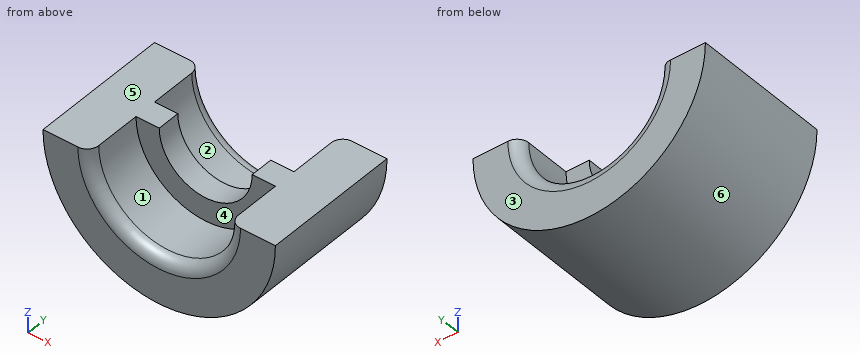
```python
from build123d import *

# Parameters (mm, degrees)
SKETCH1_W      = 1
SKETCH1_H      = 1
SKETCH1_W_2    = 2
SKETCH1_H_2    = 6
REVOLVE2_ANGLE = 180
FILLET3_R      = 0.5


with BuildPart() as part:
    # Sketch1 → Revolve2 (revolve)
    with BuildSketch(Plane.XY):
        with Locations((2.5, 0)):
            Rectangle(SKETCH1_W, SKETCH1_H)
        with Locations((4, 0)):
            Rectangle(SKETCH1_W_2, SKETCH1_H_2)
    revolve(axis=Axis((0, 0, 0), (0, 1, 0)), revolution_arc=REVOLVE2_ANGLE)

    # Fillet3
    fillet3_edges = [part.edges().sort_by_distance(p)[0] for p in [
        (0, 3, -3),
        (0, -3, -3),
    ]]
    fillet(fillet3_edges, radius=FILLET3_R)


solid = part.part
```
Can you work these out from the model? Positions are in its coordinate system, mm. Face numbers are marked on the shaded views. A direction names the side the tool comes from. Coordinates: 2 decimals unless noted, no trailing zeros. Loops run counter-clockwise (first coordinate to the right, second up) from the corner with the lowest first, then second, coordinate; pieces in that order, holes last. Notation, with made-up numbers: (76.25, -29.5) - (135.25, -29.5) arc R17 ccw to (135.25, -11.5) - close; hole circle Ø7 at (-32, 73.25). An arc over 180 degrees is marked (long way). Answer as CSV lines item,"result". Start each with the question number.
1) Thinking about a two-plate mould opening in X: for the marked faces 4, 5 and 6, which applies, pulls with the +X half, pulls with the -X half, needs draft (parallel to the pull), parting line crosses it, or undercut?
2) Suppose I cut it at A-A (x = 0). Please give me the cut outline in (y, z), plus the area to 3 significant figures.
3) For pin 1 (3 mm diameter, centred on y = -1.5, z = -2.5, fed in from +X); pin 2 (3 mm diameter, centred on x = 3.5, y = -1.5, fed in from -Z); pin 3 (2.5 mm diameter, centred on x = 1.5, z = -1.5, fed in from +Y), each with a flat end and sliding along its axis, tell me the tip position at first contact or that it passes through.
4) Which directions (+Z, -Z, +X, -X, +Y, -Y) give clear straight access to the entire face, cutting with the end or side of a thin tool? Please do the marked faces 1, 2 and 3.
5) Suppose I cut it at C-C (z = -4.5). Please give me the cut outline in (x, y), plus the area to 3 significant figures.
6) I need wall thicknesses on line 1 (Z direction, x = 0, y = 1.55); line 2 (Y direction, x = 0, z = -2.4); line 3 (Z direction, x = 4, y = 0.15). Which ranges of each line are inside material? Lowest first, please. Write a range as from..to.
7) Suppose I cut it at B-B (y = 0.3). Please give me the cut outline in (x, z), plus the area to 3 significant figures.
Check result:
1,face 4,"undercut"
1,face 5,"needs draft"
1,face 6,"parting line crosses it"
2,outline,"(-3, -5) - (3, -5) - (3, -3.5) arc R0.5 ccw to (2.5, -3) - (0.5, -3) - (0.5, -2) - (-0.5, -2) - (-0.5, -3) - (-2.5, -3) arc R0.5 ccw to (-3, -3.5) - close"
2,area,"12.9 mm²"
3,pin 1,"stops at x = 4.9"
3,pin 2,"stops at z = -4.58"
3,pin 3,"stops at y = 2.98"
4,face 1,"+Z, -Y"
4,face 2,"+Z, +Y"
4,face 3,"+Z, -Z, +X, -X, +Y"
5,outline,"(-2.18, -3) - (2.18, -3) - (2.18, 3) - (-2.18, 3) - close"
5,area,"26.2 mm²"
6,line 1,"z = -5..-3"
6,line 2,"y = -0.5..0.5"
6,line 3,"z = -3..0"
7,outline,"(-5, 0) arc R5 ccw to (5, 0) - (2, 0) arc R2 cw to (-2, 0) - close"
7,area,"33.0 mm²"
